```python
from build123d import *

# Parameters (mm, degrees)
SKETCH012_R       = 0.395
SKETCH012_R_2     = 0.46
PAD005_DEPTH      = 4
PAD005_DEPTH_BACK = 3.18
SKETCH011_W       = 3
SKETCH011_H       = 2
PAD004_DEPTH      = 4
SKETCH010_W       = 3
SKETCH010_H       = 2
PAD003_DEPTH      = 4
SKETCH_W          = 15.73
SKETCH_H          = 25
PAD_DEPTH         = 13.77
PAD001_DEPTH      = 3.18
POCKET_DEPTH      = 11.3
SKETCH004_W       = 4.6
SKETCH004_H       = 3
POCKET002_DEPTH   = 5.4
SKETCH003_W       = 6.5
SKETCH003_H       = 3
POCKET003_DEPTH   = 11.77
SKETCH005_W       = 11
SKETCH005_H       = 12
POCKET004_DEPTH   = 15.731
SKETCH009_W       = 3
SKETCH009_H       = 2
POCKET007_DEPTH   = 5
SKETCH006_W       = 16.13
SKETCH006_H       = 25.4
PAD002_DEPTH      = 13.97
SKETCH007_W       = 15.73
SKETCH007_H       = 25
POCKET005_DEPTH   = 13.7
POCKET006_DEPTH   = 0.2
SKETCH013_W       = 0.2
SKETCH013_H       = 1
PAD006_DEPTH      = 3.2
CHAMFER_SIZE      = 0.4


with BuildPart() as pins_pad:
    # Sketch012 → Pad005 (new body, two sides)
    with BuildSketch(Plane.XY) as pad005_sk:
        with Locations((-4.445, 11.43)):
            Circle(SKETCH012_R)
        with Locations((-4.445, 6.35)):
            Circle(SKETCH012_R)
        with Locations((-5.715, 8.89)):
            Circle(SKETCH012_R)
        with Locations((-3.175, 8.89)):
            Circle(SKETCH012_R)
        with Locations((3.175, 6.35)):
            Circle(SKETCH012_R)
        with Locations((5.715, 6.35)):
            Circle(SKETCH012_R)
        with Locations((0.635, 6.35)):
            Circle(SKETCH012_R)
        with Locations((1.905, 8.89)):
            Circle(SKETCH012_R)
        with Locations((4.445, 8.89)):
            Circle(SKETCH012_R)
        with Locations((2.925, 13.72)):
            Circle(SKETCH012_R_2)
        with Locations((5.465, 13.72)):
            Circle(SKETCH012_R_2)
        with Locations((-5.465, 13.72)):
            Circle(SKETCH012_R_2)
        with Locations((-2.925, 13.72)):
            Circle(SKETCH012_R_2)
    extrude(amount=PAD005_DEPTH)
    extrude(pad005_sk.sketch, amount=-PAD005_DEPTH_BACK)


with BuildPart() as led_left_green_pad:
    # Sketch011 → Pad004 (new body)
    with BuildSketch(Plane.XZ.offset(10.6)):
        with Locations((-5.55, 11.4)):
            Rectangle(SKETCH011_W, SKETCH011_H)
    extrude(amount=-PAD004_DEPTH)


with BuildPart() as led_right_yellow_pad:
    # Sketch010 → Pad003 (new body)
    with BuildSketch(Plane.XZ.offset(10.6)):
        with Locations((5.55, 11.4)):
            Rectangle(SKETCH010_W, SKETCH010_H)
    extrude(amount=-PAD003_DEPTH)


with BuildPart() as led_left_mirrored:
    # Sketch → Pad (new body)
    with BuildSketch(Plane.XY):
        with Locations((0, 1.91)):
            Rectangle(SKETCH_W, SKETCH_H)
    extrude(amount=PAD_DEPTH)

    # Sketch001 → Pad001 (new body)
    with BuildSketch(Plane(origin=(0, 0, 0), x_dir=(1, 0, 0), z_dir=(0, 0, -1))):
        Polygon((5.315, 1.445683), (5.315, 0.4), (4.269317, 0.4), (4.269317, -0.4), (5.315, -0.4), (5.315, -1.445683), (6.115, -1.445683), (6.115, -0.4), (7.160683, -0.4), (7.160683, 0.4), (6.115, 0.4), (6.115, 1.445683), align=None)
    pad001 = extrude(amount=PAD001_DEPTH)

    # Mirrored: Pad001 across Sketch001 V_Axis
    add(pad001.mirror(Plane(origin=(0, 0, 0), x_dir=(0, 0, -1), z_dir=(1, 0, 0))))

    # Sketch002 → Pocket (cut)
    with BuildSketch(Plane.XZ.offset(10.59)):
        Polygon((-6, 2), (6, 2), (6, 9.4), (3.25, 9.4), (3.25, 11), (2.15, 11), (-2.15, 11), (-3.25, 11), (-3.25, 9.4), (-6, 9.4), align=None)
    extrude(amount=-POCKET_DEPTH, mode=Mode.SUBTRACT)

    # Sketch004 → Pocket002 (cut)
    with BuildSketch(Plane.XZ.offset(10.59)):
        with Locations((0, 12.5)):
            Rectangle(SKETCH004_W, SKETCH004_H)
    extrude(amount=-POCKET002_DEPTH, mode=Mode.SUBTRACT)

    # Sketch003 → Pocket003 (cut)
    with BuildSketch(Plane.XY.offset(13.77)):
        with Locations((0, -6.69)):
            Rectangle(SKETCH003_W, SKETCH003_H)
    extrude(amount=-POCKET003_DEPTH, mode=Mode.SUBTRACT)

    # Sketch005 → Pocket004 (cut, through all)
    with BuildSketch(Plane.YZ.offset(7.865)):
        with Locations((9.5, 9)):
            Rectangle(SKETCH005_W, SKETCH005_H)
    extrude(amount=-POCKET004_DEPTH, mode=Mode.SUBTRACT)

    # Sketch009 → Pocket007 (cut)
    with BuildSketch(Plane.XZ.offset(10.59)):
        with Locations((5.55, 11.4)):
            Rectangle(SKETCH009_W, SKETCH009_H)
    pocket007 = extrude(amount=-POCKET007_DEPTH, mode=Mode.SUBTRACT)

    # Mirrored001: Pocket007 across Sketch009 V_Axis
    add(pocket007.mirror(Plane(origin=(0, -10.59, 0), x_dir=(0, -1, 0), z_dir=(1, 0, 0))), mode=Mode.SUBTRACT)


with BuildPart() as obj1:
    # Sketch006 → Pad002 (new body)
    with BuildSketch(Plane.XY):
        with Locations((0, 1.91)):
            Rectangle(SKETCH006_W, SKETCH006_H)
    extrude(amount=PAD002_DEPTH)

    # Sketch007 → Pocket005 (cut)
    with BuildSketch(Plane(origin=(0, 0, 0), x_dir=(1, 0, 0), z_dir=(0, 0, -1))):
        with Locations((0, -1.91)):
            Rectangle(SKETCH007_W, SKETCH007_H)
    extrude(amount=-POCKET005_DEPTH, mode=Mode.SUBTRACT)

    # Sketch008 → Pocket006 (cut)
    with BuildSketch(Plane.XZ.offset(10.79)):
        Polygon((-6, 2), (6, 2), (6, 9.6), (7, 10.77), (7, 12.77), (3, 12.77), (3, 13.77), (-3, 13.77), (-3, 12.77), (-7, 12.77), (-7, 10.77), (-6, 9.6), align=None)
    extrude(amount=-POCKET006_DEPTH, mode=Mode.SUBTRACT)

    # Sketch013 → Pad006 (new body)
    with BuildSketch(Plane(origin=(0, 0, 0), x_dir=(1, 0, 0), z_dir=(0, 0, -1))):
        with Locations((7.965, -3.05)):
            Rectangle(SKETCH013_W, SKETCH013_H)
    pad006 = extrude(amount=PAD006_DEPTH)

    # Mirrored002: Pad006 across Sketch013 V_Axis
    add(pad006.mirror(Plane(origin=(0, 0, 0), x_dir=(0, 0, -1), z_dir=(1, 0, 0))))

    # Chamfer
    chamfer_edges = [obj1.edges().sort_by_distance(p)[0] for p in [
        (7.965, 3.55, -3.2),
        (7.965, 2.55, -3.2),
        (-7.965, 2.55, -3.2),
        (-7.965, 3.55, -3.2),
    ]]
    chamfer(chamfer_edges, length=CHAMFER_SIZE)

    # Fusion: union Pins_Pad, LED_Left_Green_Pad, LED_Right_Yellow_Pad, LED_Left_Mirrored
    add(pins_pad.part)
    add(led_left_green_pad.part)
    add(led_right_yellow_pad.part)
    add(led_left_mirrored.part)


solid = obj1.part
```
For this review, take the finished solid that the model builds, in its own axes (mm). A direction names the side the tool comes from. Coordinates: 2 decimals unless noted, no trailing zeros. Order: outer loops, then holes, each group sorted by start corner. A loop starts at its lowest first (then second) coordinate and runs counter-clockwise, first axis right, second up. Notation, with made-up numbers: (-13.5, 30.5) -> (6.5, 30.5) arc R20 ccw to (6.5, 62.5) -> close; hole circle Ø5 at (6, 79). An arc over 180 degrees is marked (long way). Use CSV: the item, a comma, the result in double quotes. Start each with the question number.
Item 1: Draft analysis for pull direction X (two halves, no side actions). For faces 1 (the face through (-2.985, 14.176, 3.507)), 2 (the face through (-3, 14, -3.18)), 3 (the face through (-8.065, 2, 7)), state which applies: pulls with the +X half, pulls with the -X half, needs draft (parallel to the pull), parting line crosses it, or undercut.
Item 2: Insertion check: pin 1 (0.8 mm diameter, centred on y = -1, z = -2, fed in from +X) (3 decimals); pin 2 (0.5 mm diameter, centred on x = -2.5, y = -9.5, fed in from -Z); pin 3 (0.8 mm diameter, centred on x = -0.5, z = 12, fed in from -Y). Each pin has a flat end and moves straight along its axis. Give the tip position at first contact, or say it passes through.
Item 3: Wall thickness on probe 1 along X at (y, z) = (-4, 9) (3 decimals); probe 2 along Z at (x, y) = (0.75, 9); probe 3 along X at (y, z) = (8, 11.5) (3 decimals): over which ranges is each line inside the solid? List them lowest first.
Item 4: We need section D-D, the plane z = -0.5. Give the number of separate pieces and of enclosed holes in the cut face, then the cut area to 3 significant figures.
Item 5: We need section B-B, the plane y = 5.5. Give the boundary of the cut face in (x, z) (3 decimals), then the cut area to 3 significant figures.
Item 6: We need section A-A, the plane z = 5.5. Give the boundary of the cut face in (x, y) (3 decimals).
Item 7: We need section C-C, the plane y = -2.5. Give the boundary of the cut face in (x, z) (3 decimals).
Item 8: For faces 4 (the face through (3, -9, 11)), 5 (the face through (6.115, 1, -2)), 6 (the face through (2.865, 14.176, 3.507)), list the 3-axis set-ups (+Z, -Z, +X, -X, +Y, -Y) from which the entire face can be reached by the end or side of a thin tool; tool diameter is ignored.
Derived:
1,face 1,"undercut"
1,face 2,"needs draft"
1,face 3,"pulls with the -X half"
2,pin 1,"stops at x = 6.115"
2,pin 2,"stops at z = 0"
2,pin 3,"stops at y = -5.19"
3,probe 1,"x = -8.065 to -6, 6 to 8.065"
3,probe 2,"z = 0 to 3, 13.7 to 13.97"
3,probe 3,"x = -8.065 to -7.865, 7.865 to 8.065"
4,separate pieces,"17"
4,enclosed holes,"0"
4,area,"15.4 mm^2"
5,outline,"(-8.065, 0) -> (8.065, 0) -> (8.065, 13.97) -> (-8.065, 13.97) -> close; hole (-7.865, 3) -> (7.865, 3) -> (7.865, 13.7) -> (-7.865, 13.7) -> close"
5,area,"57.0 mm^2"
6,outline,"(-8.065, -10.79) -> (-6, -10.79) -> (-6, 0.71) -> (6, 0.71) -> (6, -10.79) -> (8.065, -10.79) -> (8.065, 14.61) -> (-8.065, 14.61) -> close; hole (-7.865, 4) -> (7.865, 4) -> (7.865, 14.41) -> (-7.865, 14.41) -> close"
7,outline,"(-8.065, 0) -> (8.065, 0) -> (8.065, 13.97) -> (-8.065, 13.97) -> close; hole (-6, 2) -> (6, 2) -> (6, 9.4) -> (3.25, 9.4) -> (3.25, 11) -> (-3.25, 11) -> (-3.25, 9.4) -> (-6, 9.4) -> close"
8,face 4,"-Y"
8,face 5,"-Z, +X, +Y"
8,face 6,"none"
